Input: part model. Units: mm. Frame: model coordinates. Face numbers are marked on the shaded views. A direction names the side the tool comes from. Coordinates: 2 decimals unless noted, no trailing zeros. Loops run counter-clockwise (first coordinate to the right, second up) from the corner with the lowest first, then second, coordinate; pieces in that order, holes last. Notation, with made-up numbers: (48.25, -12) -> (60.25, -12) arc R22 cw to (60.25, 11) -> close; hole circle Ø4 at (-2.5, 16). An arc over 180 degrees is marked (long way). Answer as a JSON object with one key per item and string values.
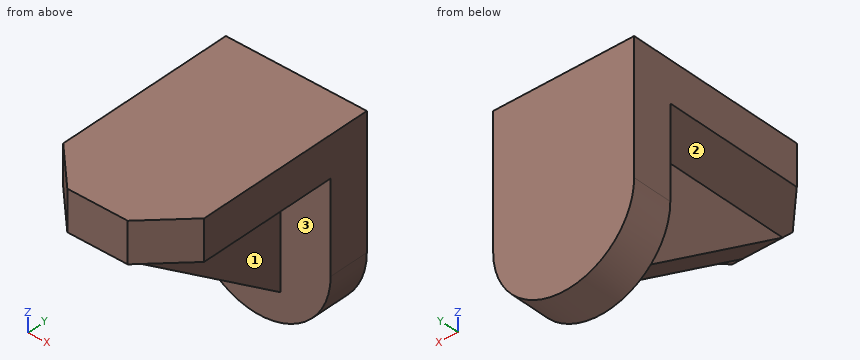
from build123d import *

# Parameters (mm, degrees)
BOSS_EXTRUDE2_DEPTH = 12
BOSS_EXTRUDE4_DEPTH = 12
RIB1_REACH          = 81.189
SKETCH7_WALLS_W     = 12
SKETCH7_WALLS_H     = 226.916782225


with BuildPart() as part:
    # Sketch1 → Boss-Extrude2 (new body)
    with BuildSketch(Plane.XY):
        Polygon((-31.541899517, 54.96059397), (-31.541899517, 0.96059397), (-19.541899517, -11.03940603), (-1.541899517, -11.03940603), (10.458100483, 0.96059397), (10.458100483, 54.96059397), align=None)
    extrude(amount=BOSS_EXTRUDE2_DEPTH)

    # Sketch2 → Boss-Extrude4 (add)
    with BuildSketch(Plane(origin=(0, 54.96059397, 0), x_dir=(1, 0, 0), z_dir=(0, 1, 0))):
        with BuildLine():
            Line((10.458100483, 0), (10.458100483, 27))
            ThreePointArc((10.458100483, 27), (-10.541899517, 48), (-31.541899517, 27))
            Line((-31.541899517, 27), (-31.541899517, 0))
            Line((-31.541899517, 0), (10.458100483, 0))
        make_face()
    extrude(amount=-BOSS_EXTRUDE4_DEPTH)

    # Sketch7 walls → Rib1 (add, up to next)
    with BuildSketch(Plane(origin=(0, -3.746614572, -5.227167373), x_dir=(1, 0, 0), z_dir=(0, 0.5825680402279159, 0.8127819378560314)), mode=Mode.PRIVATE) as rib1_sk1:
        with Locations((-10.541899517, 24.296475579)):
            Rectangle(SKETCH7_WALLS_W, SKETCH7_WALLS_H)
    rib1_tool1 = extrude(rib1_sk1.sketch, amount=RIB1_REACH, mode=Mode.PRIVATE) - part.part
    add(rib1_tool1.solids().sort_by_distance((-10.541899517, 16.001121931, -19.381517535))[0])


solid = part.part
1. Section query D-D (z = -20). Return loops of the section in (x, y), plus the area to 3 significant figures.
Reply:
{"outline": "(-31.54, 42.96) -> (-16.54, 42.96) -> (-16.54, 16.86) -> (-4.54, 16.86) -> (-4.54, 42.96) -> (10.46, 42.96) -> (10.46, 54.96) -> (-31.54, 54.96) -> close", "area": "817 mm2"}
2. Section query B-B (y = 7.5). Return loops of the section in (x, z).
Reply:
{"outline": "(-31.54, 0) -> (-16.54, 0) -> (-16.54, -13.29) -> (-4.54, -13.29) -> (-4.54, 0) -> (10.46, 0) -> (10.46, 12) -> (-31.54, 12) -> close"}
3. Line query: line 1 along Z through (x, y) = (0.5, 19); line 2 along Y through (x, z) = (-24, -14.5); line 3 along X through (y, z) = (33, -21). Output: solid intervals per line, ascending.
Reply:
{"line 1": "z = 0 to 12", "line 2": "y = 42.96 to 54.96", "line 3": "x = -16.54 to -4.54"}
4. Access query for the marked faces 1, 2 and 3. Directions: +Z, -Z, +X, -X, +Y, -Y. A direction counts if a zero-diameter tool reaches every point of the face in a straight line with its end or side. Return the directions, or none.
Reply:
{"face 1": "-Z, +X, -Y", "face 2": "-Z, -X, -Y", "face 3": "-Z, -Y"}
5. Section query A-A (z = 3). Return loops of the section in (x, y), plus the area to 3 significant figures.
Reply:
{"outline": "(-31.54, 0.96) -> (-19.54, -11.04) -> (-1.54, -11.04) -> (10.46, 0.96) -> (10.46, 54.96) -> (-31.54, 54.96) -> close", "area": "2,630 mm2"}
6. Section query C-C (x = -9). Return loops of the section in (y, z), plus the area to 3 significant figures.
Reply:
{"outline": "(-11.04, 0) -> (42.96, -38.7) -> (42.96, -47.94) -> (54.96, -47.94) -> (54.96, 12) -> (-11.04, 12) -> close", "area": "2,410 mm2"}
7. Pin query (flat end, axial travel): P1, Ø2, axis at y = 44.5, z = -37.5, coming from the +X side; P2, Ø12, axis at y = 13, z = -24, coming from the -X side; P3, Ø1.5, axis at y = 18.5, z = -24.5, coming from the +X side; P4, Ø12.5, axis at x = -8.5, z = -12.5, coming from the -Y side. Return the tip coordinate at first contact, or that it passes through.
Reply:
{"P1": "stops at x = 8.19", "P2": "stops at x = -16.54", "P3": "passes through", "P4": "stops at y = -2.32"}
